Check sheet for the modelled part. Datum: model origin and axes. Units: mm. A direction names the side the tool comes from. Give positions to 0.01 mm unless a question says otherwise; leave off trailing zeros. Write each loop counter-clockwise with the first axis right and the second up, starting at its lowest first coordinate (ties: lowest second). Pieces come first, ordered by that corner, then holes. Notation, with made-up numbers: (48.5, -20) -> (61.5, -20) arc R29 cw to (61.5, 19) -> close; hole circle Ø7 at (-32, -28). An arc over 180 degrees is marked (long way). Answer as a JSON object with one key per item and string values.
Autodesk Inventor part; units mm, degrees
ref_plane "YZ Plane" through (0, 0, 0) normal (1, 0, 0) x (0, 1, 0)
ref_plane "XZ Plane" through (0, 0, 0) normal (0, 1, 0) x (-1, 0, 0)
ref_plane "XY Plane" through (0, 0, 0) normal (0, 0, 1) x (1, 0, 0)
sketch "Sketch1" plane through (0, 0, 0) normal (0, 0, 1) x (1, 0, 0)
  line L0 (-24.6776, 0) -> (23.5544, 0)
  line L1 (0, -22.6406) -> (0, 25.7747)
  circle A0 centre (-13.5, 0) radius 1.15
  circle A1 centre (-13.5, 0) radius 2.35
  circle A2 centre (13.5, 0) radius 1.15
  circle A3 centre (13.5, 0) radius 2.35
  circle A4 centre (0, 6) radius 1
  circle A5 centre (0, 6) radius 0.5
  circle A6 centre (0, -10.75) radius 1.25
  circle A7 centre (-8.5, 8.5) radius 1.25
  circle A8 centre (8.5, 8.5) radius 1.25
  line L2 (-11.6, -3.6) -> (-11.25, -3.6)
  line L3 (-11.25, -3.6) -> (-11.25, -4.1)
  line L4 (-11.25, -4.1) -> (-11.6, -4.1)
  line L5 (-11.6, -4.1) -> (-11.6, -3.6)
  line L6 (11.25, -4.1) -> (11.25, -3.6)
  line L7 (11.25, -3.6) -> (11.6, -3.6)
  line L8 (11.6, -3.6) -> (11.6, -4.1)
  line L9 (11.6, -4.1) -> (11.25, -4.1)
  line L10 (-11.6, 3.6) -> (-11.6, 4.1)
  line L11 (-11.6, 4.1) -> (-11.25, 4.1)
  line L12 (-11.25, 4.1) -> (-11.25, 3.6)
  line L13 (-11.25, 3.6) -> (-11.6, 3.6)
  line L14 (11.25, 3.6) -> (11.25, 4.1)
  line L15 (11.25, 4.1) -> (11.6, 4.1)
  line L16 (11.6, 4.1) -> (11.6, 3.6)
  line L17 (11.6, 3.6) -> (11.25, 3.6)
  arc A9 (14.8788, 1.903) -> (4.6837, 14.25) centre (0, 0) ccw
  arc A10 (4.6837, 14.25) -> (-14.8788, 1.903) centre (0, 0) ccw
  arc A11 (4.6837, -14.25) -> (14.8788, -1.903) centre (0, 0) ccw
  circle A12 centre (5.4353, -14.25) radius 0.1148
  line L18 (-4.6837, -14.25) -> (4.6837, -14.25)
  arc A13 (14.8788, 1.903) -> (-14.8788, 1.903) centre (0, 0) ccw
  arc A14 (-14.8788, -1.903) -> (-14.5616, -3.6) centre (0, 0) ccw
  arc A15 (-14.5616, -3.6) -> (-4.6837, -14.25) centre (0, 0) ccw
  arc A16 (-14.5616, 3.6) -> (-14.8788, 1.903) centre (0, 0) ccw
  arc A17 (0, 15) -> (-14.5616, 3.6) centre (0, 0) ccw
  arc A18 (-14.5616, 3.6) -> (-14.8788, 1.903) centre (0, 0) ccw
  point P0 (-15.6415, -0.9678)
  point P1 (0, -15.6714)
  point P2 (15.1605, -1.6629)
  dimension "d2" = 2.3
  dimension "d3" = 4.7
  dimension "d4" = 13.5
  dimension "d7" = 360
  dimension "d9" = 2
  dimension "d10" = 1
  dimension "d11" = 6
  dimension "d12" = 2.5
  dimension "d13" = 10.75
  dimension "d14" = 19.25
  dimension "d16" = 8.5
  dimension "d17" = 0.35
  dimension "d18" = 0.5
  dimension "d19" = 11.25
  dimension "d20" = 3.6
  dimension "d23" = 22.85
  dimension "d26" = 7.7
  dimension "d48" = 14.25
extrude "Extrusion1" add sketch "Sketch1" along normal blind 7 contours A0 L0 A1 | L0 A1 A0 | A1 A10 L1 A4 L0 | L0 L1 A6 L18 A15 A14 A1 | L1 A4 A10 A9 A3 L0 | L0 A3 A11 L18 L1 A6 | A3 L0 A2 | L0 A2 A3 | A6 L1 | L1 A6 | A4 L1 A5 | L1 A5 A4 | A5 L1 | L1 A5 | A7 | A8 | L2 L3 L4 L5 | L6 L7 L8 L9 | L10 L11 L12 L13 | L14 L15 L16 L17
sketch "Sketch2" plane through (0, 0, 0) normal (0, 0, -1) x (-1, 0, 0)
  point P0 (0, 0)
extrude "Extrusion2" add sketch "Sketch1" against normal blind 3 contours A6 L1 | L1 A6 | A7 | A8
fillet "Fillet1" radius 0.5 3 edges at (7.25, 8.5, -3) (-1.25, -10.75, -3) (-9.75, 8.5, -3)
extrude "Extrusion3" add sketch "Sketch1" against normal blind 10.95 contours A5 L1 | L1 A5
extrude "Extrusion4" add sketch "Sketch1" against normal blind 2.3 contours A4 L1 A5 | L1 A5 A4
extrude "Extrusion5" add sketch "Sketch1" against normal blind 2.8 contours L2 L3 L4 L5 | L6 L7 L8 L9 | L10 L11 L12 L13 | L14 L15 L16 L17
extrude "Extrusion6" cut sketch "Sketch1" along normal blind 0.3 contours A1 A10 L1 A4 L0 | L0 L1 A6 L18 A15 A14 A1 | L1 A4 A10 A9 A3 L0 | L0 A3 A11 L18 L1 A6
equation "\"d23\" = 2 * d19 + d17"
equation "\"d26\" = 2 * d20 + d18"
properties part number "VID26" material "PBT Plastic"
1. Sectioned sample at D-D, the plane y = -10.75. Enter the section's corners in (x, z), plus the area to 3 significant figures.
Determined:
{"outline": "(-10.46, 0.3) -> (-1.25, 0.3) -> (-1.25, -2.5) arc R0.5 ccw to (-0.75, -3) -> (0.75, -3) arc R0.5 ccw to (1.25, -2.5) -> (1.25, 0.3) -> (10.46, 0.3) -> (10.46, 7) -> (-10.46, 7) -> close", "area": "148 mm^2"}
2. Sectioned sample at A-A, the plane y = 0. Enter the section's corners in (x, z).
Determined:
{"outline": "(-15.85, 0) -> (-14.65, 0) -> (-14.65, 7) -> (-15.85, 7) -> close; (-12.35, 0) -> (-11.15, 0) -> (-11.15, 0.3) -> (11.15, 0.3) -> (11.15, 0) -> (12.35, 0) -> (12.35, 7) -> (-12.35, 7) -> close; (14.65, 0) -> (15.85, 0) -> (15.85, 7) -> (14.65, 7) -> close"}
3. Mould release check, pull along Y, two halves, no side actions. Record for faces 3 (the face through (-0.16, -9.51, -1.08)), 4 (the face through (8.5, 8.5, -3)), 5 (the face through (-14.74, -2.77, 3.6)): released by +Y, released by -Y, zero draft, split by the parting line, or undercut.
Determined:
{"face 3": "undercut", "face 4": "zero draft", "face 5": "released by -Y"}
4. Go/stop test with flat-tipped pins: P1, Ø1.4, axis at x = -13.5, y = 0, coming from the -Z side; P2, Ø2, axis at y = 5, z = 2, coming from the -X side; P3, Ø1.6, axis at x = -8, y = 8.5, coming from the -Z side; P4, Ø6, axis at y = 3, z = -1, coming from the -X side. Record where each tip stops, or that it passes through.
Determined:
{"P1": "through", "P2": "x = -14.46", "P3": "z = -3", "P4": "x = -15.84"}
5. Access from +Z, -Z, +X, -X, +Y, -Y to the whole of each face (thin tool, end or side, straight path). Record for faces 1 (the face through (-9.75, 8.55, -1.08)), 2 (the face through (12, -9, 4)).
Determined:
{"face 1": "-Z", "face 2": "+Z, -Z, +X, -Y"}
6. Sectioned sample at C-C, the plane x = 13.5. Enter the section's corners in (y, z), plus the area to 3 significant figures.
Determined:
{"outline": "(-6.54, 0.3) -> (-2.35, 0.3) -> (-2.35, 0) -> (-1.15, 0) -> (-1.15, 7) -> (-6.54, 7) -> close; (1.15, 0) -> (2.35, 0) -> (2.35, 0.3) -> (6.54, 0.3) -> (6.54, 7) -> (1.15, 7) -> close", "area": "72.9 mm^2"}
7. Sectioned sample at B-B, the plane z = 4.75. Enter the section's corners in (x, y).
Determined:
{"outline": "(-14.88, -1.9) arc R15 ccw to (-14.56, -3.6) arc R15 ccw to (-4.68, -14.25) -> (4.68, -14.25) arc R15 ccw to (14.88, -1.9) arc R2.35 ccw to (14.88, 1.9) arc R15 ccw to (4.68, 14.25) arc R15 ccw to (-14.88, 1.9) arc R2.35 ccw to start; hole circle Ø2.3 at (-13.5, 0); hole circle Ø2.3 at (13.5, 0)"}
8. Scan lines: L1, parallel to X at y = 0, z = 4.75; L2, parallel to Y at x = 11.5, z = -0.75; L3, parallel to X at y = 1, z = 1.25. Record each from-to range of solid material in increasing order. Write a range as [from, to].
Determined:
{"L1": "[-15.85, -14.65], [-12.35, 12.35], [14.65, 15.85]", "L2": "[-4.1, -3.6], [3.6, 4.1]", "L3": "[-15.63, -14.07], [-12.93, 12.93], [14.07, 15.63]"}
